Could you check a few things on this model? Use its own coordinates, in mm. A direction names the side the tool comes from. Coordinates: 2 decimals unless noted, no trailing zeros. Loops run counter-clockwise (first coordinate to the right, second up) from the corner with the lowest first, then second, coordinate; pieces in that order, holes last. Notation, with made-up numbers: (86, 27) - (102, 27) arc R35 cw to (102, 59) - close; hole circle Ø2 at (-5.75, 57.25). An arc over 180 degrees is marked (long way). One line per question, with ' | ' between items. Start each with the question number.
1. I want a section at D-D, the plane x = 24.5. Write out the boundary of the cut face in (y, z), then the cut area to 3 significant figures.
2. I want a section at B-B, the plane z = 13.75. Write out the boundary of the cut face in (x, y).
3. I'm going to push flat-ended pins straight in: P1, Ø4, axis at x = 10, y = 17.5, coming from the +Z side; P2, Ø5, axis at x = 16.1, y = 30.76, coming from the +Z side. Where does each tip first touch, or does it pass through?
4. Which directions (+Z, -Z, +X, -X, +Y, -Y) give clear straight access to the entire face, cutting with the end or side of a thin tool? Please do faces 5 (the flat face through (5, 13, 12.947)), 6 (the cylindrical face through (-4.4, 10.83, 0.57)), 7 (the cylindrical face through (4.285, 22.812, 4.93)).
5. I want a section at C-C, the plane y = -2.5. Write out the boundary of the cut face in (x, z).
6. Please list where these lines run through material, in increasing order: L1, parallel to X at y = 31.5, z = 10.5; L2, parallel to Y at x = 23.5, z = 11; L3, parallel to Y at x = 8, z = 7.25. Write a range as [from, to].
7. We'd pull the mould along X, two halves only. Please class faces 1 (the cylindrical face through (29.4, 35.43, 8.38)), 2 (the cylindrical face through (2.286, 15.989, 4.93)), 3 (the cylindrical face through (8.1, 34, 8.9)), 4 (the cylindrical face through (12.28, -14.4, 0.57)): pulls with the +X half, pulls with the -X half, needs draft (parallel to the pull), parting line crosses it, or undercut.
8. I want a section at A-A, the plane y = 16. Write out the boundary of the cut face in (x, z), then the cut area to 3 significant figures.
Autodesk Inventor part; units mm, degrees
ref_plane "YZ Plane" through (0, 0, 0) normal (1, 0, 0) x (0, 1, 0)
ref_plane "XZ Plane" through (0, 0, 0) normal (0, 1, 0) x (-1, 0, 0)
ref_plane "XY Plane" through (0, 0, 0) normal (0, 0, 1) x (1, 0, 0)
ref_plane "Arbeitsebene1" through (0, 0, 0) normal (0, 0, 1) x (1, 0, 0)
sketch "Skizze1" plane through (0, 0, 0) normal (0, 0, 1) x (1, 0, 0)
  line L0 (20, 36) -> (0, 36)
  line L1 (0, 0) -> (0, 36)
  line L2 (20, 0) -> (0, 0)
  line L3 (20, 0) -> (20, 36)
  arc A0 (15.4309, 14.7711) -> (15.4309, 17.2289) centre (16.1016, 16) ccw
  arc A1 (15.4309, 17.2289) -> (15.4309, 14.7711) centre (8.2858, 16) ccw
  circle A2 centre (8.2858, 30.7551) radius 1.4
  circle A3 centre (16.1016, 30.7551) radius 1.4
  circle A4 centre (8.2858, 16) radius 6
  line L4 (14.1858, 12.5359) -> (8.3358, 9.1584)
  line L5 (2.3358, 12.6225) -> (2.3358, 19.3775)
  line L6 (8.3358, 22.8416) -> (14.1858, 19.4641)
  circle A5 centre (8.2858, 16) radius 5.95
  arc A6 (14.1858, 12.5359) -> (14.1858, 19.4641) centre (12.1858, 16) ccw
  arc A7 (2.3358, 12.6225) -> (8.3358, 9.1584) centre (6.3358, 12.6225) ccw
  arc A8 (8.3358, 22.8416) -> (2.3358, 19.3775) centre (6.3358, 19.3775) ccw
  line L7 (-5, 36) -> (30, 36)
  line L8 (30, 36) -> (30, -15)
  line L9 (30, -15) -> (-5, -15)
  line L10 (-5, -15) -> (-5, 36)
  point P0 (20.1858, 16)
  point P1 (2.3358, 5.6943)
  point P2 (2.3358, 26.3057)
  point P3 (10.5914, 21.5393)
  point P4 (11.9302, 20.7664)
  point P5 (11.9302, 11.2336)
  point P6 (10.5914, 10.4607)
  point P7 (2.3358, 15.227)
  point P8 (2.3358, 16.773)
  dimension "d0" = 11.9
  dimension "d1" = 4
  dimension "d2" = 10
  dimension "d3" = 0
  dimension "d4" = 5
  dimension "d5" = 15
extrude "Extrusion1" add sketch "Skizze1" along normal blind 10 contours L3 L2 L1 L0 | L7 L8 L9 L10 L1 L2 L3 | A6 A0 | A1 A7 L4 A4 A6 | A6 L6 A4 A8 A1 | A1 A8 L5 A4 A7
sketch "Skizze2" plane through (0, 0, 10) normal (0, 0, 1) x (1, 0, 0)
  line L0 (-5, -15) -> (30, -15)
  line L1 (30, -15) -> (30, 36)
  line L2 (30, 36) -> (-5, 36)
  line L3 (-5, 36) -> (-5, -15)
  circle A0 centre (16.1016, 30.7551) radius 1.4
  circle A1 centre (8.2858, 30.7551) radius 1.4
  arc A2 (8.3358, 22.8416) -> (2.3358, 19.3775) centre (6.3358, 19.3775) ccw
  line L4 (8.3358, 22.8416) -> (10.5914, 21.5393)
  arc A3 (11.9302, 20.7664) -> (10.5914, 21.5393) centre (8.2858, 16) ccw
  line L5 (11.9302, 20.7664) -> (14.1858, 19.4641)
  arc A4 (14.1858, 12.5359) -> (14.1858, 19.4641) centre (12.1858, 16) ccw
  line L6 (14.1858, 12.5359) -> (11.9302, 11.2336)
  arc A5 (10.5914, 10.4607) -> (11.9302, 11.2336) centre (8.2858, 16) ccw
  line L7 (10.5914, 10.4607) -> (8.3358, 9.1584)
  arc A6 (2.3358, 12.6225) -> (8.3358, 9.1584) centre (6.3358, 12.6225) ccw
  line L8 (2.3358, 12.6225) -> (2.3358, 15.227)
  arc A7 (2.3358, 16.773) -> (2.3358, 15.227) centre (8.2858, 16) ccw
  line L9 (2.3358, 16.773) -> (2.3358, 19.3775)
  circle A8 centre (8.2858, 16) radius 3.9
  point P0 (0, 0)
  dimension "d8" = 7.8
extrude "Extrusion2" add sketch "Skizze2" along normal up to surface (2.9472 mm away) contours L3 L2 L1 L0 | L4 A3 L5 A4 L6 A5 L7 A6 L8 A7 L9 A2
sketch "Skizze3" plane through (0, 0, 12.9472) normal (0, 0, 1) x (1, 0, 0)
  circle A0 centre (8.2858, 16) radius 3.6158
  line L0 (4.0358, 12) -> (4.0358, 20)
  line L1 (12.5358, 20) -> (12.5358, 12)
  line L2 (4.0358, 20.25) -> (12.5358, 20.25)
  line L3 (12.5358, 20.25) -> (12.5358, 11.75)
  line L4 (12.5358, 11.75) -> (4.0358, 11.75)
  line L5 (4.0358, 11.75) -> (4.0358, 20.25)
  line L6 (4.0358, 20.25) -> (12.5358, 11.75) construction
  line L7 (12.5358, 20.25) -> (4.0358, 11.75) construction
  line L8 (30, -15) -> (30, 36)
  line L9 (30, 36) -> (-5, 36)
  line L10 (-5, 36) -> (-5, -15)
  line L11 (-5, -15) -> (30, -15)
  circle A1 centre (8.2858, 16) radius 3.9
  circle A2 centre (8.2858, 30.7551) radius 1.4
  circle A3 centre (16.1016, 30.7551) radius 1.4
  point P0 (0, 0)
  point P1 (11.389, 20.2649)
  dimension "d11" = 8.5
  dimension "d12" = 8.5
extrude "Extrusion3" add sketch "Skizze3" along normal blind 2 contours L11 L10 L9 L8 | A3
sketch "Skizze4" plane through (0, 0, 14.9472) normal (0, 0, 1) x (1, 0, 0)
  circle A0 centre (8.2858, 30.7551) radius 1.4
  circle A1 centre (16.1016, 30.7551) radius 1.4
  arc A2 (21.7732, 26.3966) -> (20.7732, 27.3966) centre (20.7732, 26.3966) ccw
  arc A3 (20.7732, -12.6034) -> (21.7732, -11.6034) centre (20.7732, -11.6034) ccw
  circle A4 centre (26.449, 23.3562) radius 1.4
  circle A5 centre (26.449, -4.8113) radius 1.4
  point P0 (0, 0)
  dimension "d23" = 2.8
  dimension "d24" = 2.8
hole "Bohrung1" at (8.2858, 30.7551, 14.9472) at (16.1016, 30.7551, 14.9472) at (26.449, 23.3562, 14.9472) at (26.449, -4.8113, 14.9472) direction (0, 0, -1) diameter 2.8 depth 30 counterbore diameter 6.5 counterbore depth 12
fillet "Rundung1" radius 2 8 edges at (-5, -15, 7.4736) (-5, 36, 7.4736) (30, 36, 7.4736) (30, 10.5, 0) (12.5, -15, 0) (-5, 10.5, 0) (12.5, 36, 0) (30, -15, 7.4736)
properties part number "30_ESP32_Camera_tray"
Results are:
1) outline: (-15, 2) arc R2 ccw to (-13, 0) - (34, 0) arc R2 ccw to (36, 2) - (36, 14.95) - (25.96, 14.95) - (25.96, 2.95) - (20.76, 2.95) - (20.76, 14.95) - (-2.21, 14.95) - (-2.21, 2.95) - (-7.41, 2.95) - (-7.41, 14.95) - (-15, 14.95) - close | area: 636 mm2
2) outline: (-5, -13) arc R2 ccw to (-3, -15) - (28, -15) arc R2 ccw to (30, -13) - (30, 34) arc R2 ccw to (28, 36) - (-3, 36) arc R2 ccw to (-5, 34) - close; hole (4.04, 11.75) - (12.54, 11.75) - (12.54, 20.25) - (4.04, 20.25) - close; hole circle Ø6.5 at (8.29, 30.76); hole circle Ø6.5 at (16.1, 30.76); hole circle Ø6.5 at (26.45, -4.81); hole circle Ø6.5 at (26.45, 23.36)
3) P1: stops at z = 12.95 | P2: stops at z = 2.95
4) face 5: +Z | face 6: -Z, -X, +Y, -Y | face 7: -Z
5) outline: (-5, 2) arc R2 ccw to (-3, 0) - (28, 0) arc R2 ccw to (30, 2) - (30, 14.95) - (28.73, 14.95) - (28.73, 2.95) - (24.16, 2.95) - (24.16, 14.95) - (-5, 14.95) - close
6) L1: x = [-5, 5.12], [11.45, 12.94], [19.27, 30] | L2: y = [-15, -6.18], [-3.45, 21.99], [24.72, 36] | L3: y = [-15, 8.99], [23.01, 27.52], [33.99, 36]
7) face 1: pulls with the +X half | face 2: undercut | face 3: undercut | face 4: needs draft
8) outline: (-5, 2) arc R2 ccw to (-3, 0) - (2.29, 0) - (2.29, 10) - (4.39, 10) - (4.39, 12.95) - (4.04, 12.95) - (4.04, 14.95) - (-5, 14.95) - close; (12.19, 10) - (16.19, 10) - (16.19, 0) - (28, 0) arc R2 ccw to (30, 2) - (30, 14.95) - (12.54, 14.95) - (12.54, 12.95) - (12.19, 12.95) - close | area: 342 mm2
